For this review, use the dimensioned drawing (mm, ordinates from the lowest corner) and the shaded views. Coordinates: 2 decimals unless noted, no trailing zeros. Order: outer loops, then holes, each group sorted by start corner. A loop starts at its lowest first (then second) coordinate and runs counter-clockwise, first axis right, second up. Notation, with made-up numbers: M 70.25,57.5 L 115.25,57.5 A26 cw 115.25,96.5 Z; hole C 82.25,5.5 d10. An arc over 180 degrees is marked long. Write each question's results on one line, items separated by ' | '.
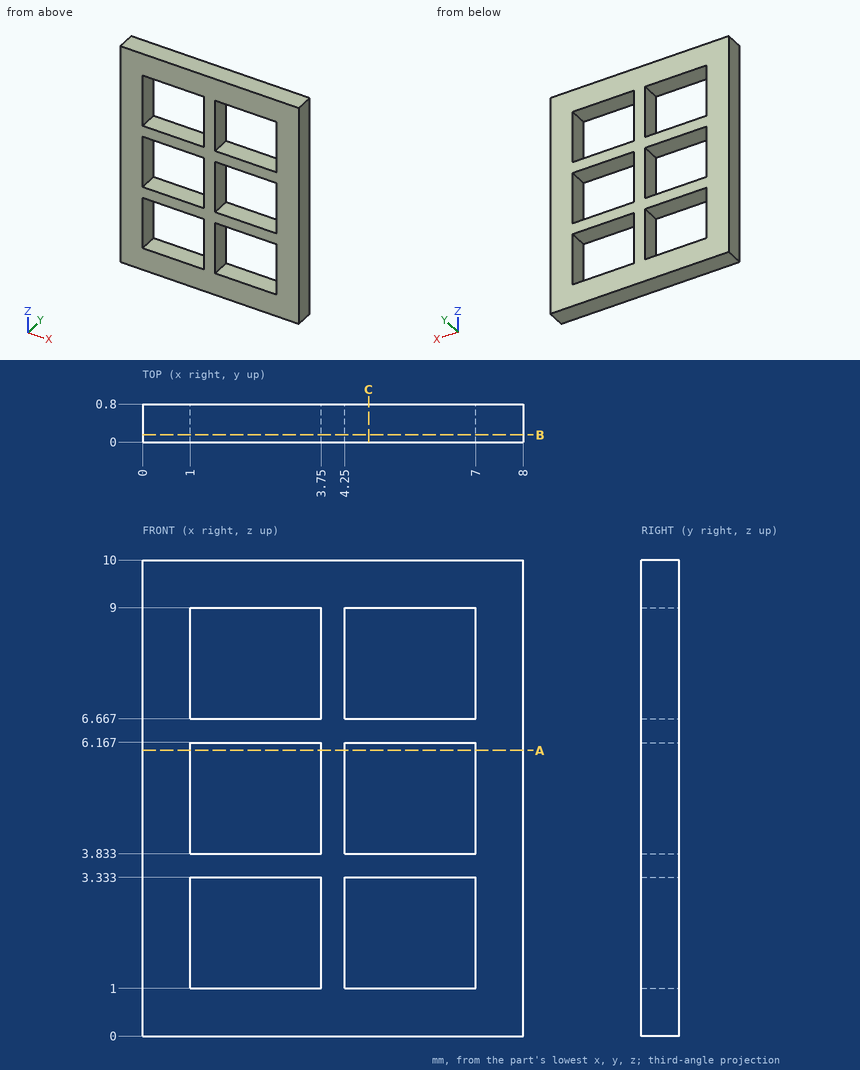
1) To check wall thickness, follow line 1 along Z through (x, y) = (5.5, 0.6); line 2 along X through (y, z) = (0.15, 5). State the ranges of each line that lie inside material, in increasing order.
Solutions:
line 1: 0 to 1, 3.33 to 3.83, 6.17 to 6.67, 9 to 10 | line 2: 0 to 1, 3.75 to 4.25, 7 to 8
2) Take a section at A-A on z = 6. State the section outline as (x, y) points.
Solutions:
outline: M 0,0 L 1,0 L 1,0.8 L 0,0.8 Z; M 3.75,0 L 4.25,0 L 4.25,0.8 L 3.75,0.8 Z; M 7,0 L 8,0 L 8,0.8 L 7,0.8 Z
3) Take a section at B-B on y = 0.15. State the section outline as (x, z) points.
Solutions:
outline: M 0,0 L 8,0 L 8,10 L 0,10 Z; hole M 1,1 L 3.75,1 L 3.75,3.33 L 1,3.33 Z; hole M 1,3.83 L 3.75,3.83 L 3.75,6.17 L 1,6.17 Z; hole M 1,6.67 L 3.75,6.67 L 3.75,9 L 1,9 Z; hole M 4.25,1 L 7,1 L 7,3.33 L 4.25,3.33 Z; hole M 4.25,3.83 L 7,3.83 L 7,6.17 L 4.25,6.17 Z; hole M 4.25,6.67 L 7,6.67 L 7,9 L 4.25,9 Z
4) Take a section at C-C on x = 4.75. State the section outline as (y, z) points.
Solutions:
outline: M 0,0 L 0.8,0 L 0.8,1 L 0,1 Z; M 0,3.33 L 0.8,3.33 L 0.8,3.83 L 0,3.83 Z; M 0,6.17 L 0.8,6.17 L 0.8,6.67 L 0,6.67 Z; M 0,9 L 0.8,9 L 0.8,10 L 0,10 Z
